Check sheet for the modelled part. Datum: model origin and axes. Units: mm. Face numbers are marked on the shaded views. A direction names the side the tool comes from. Coordinates: 2 decimals unless noted, no trailing zeros. Loops run counter-clockwise (first coordinate to the right, second up) from the corner with the lowest first, then second, coordinate; pieces in that order, holes last.
from build123d import *

# Parameters (mm, degrees)
SKETCH_1_R               = 25
SKETCH_1_R_2             = 1.5
EXTRUDE_1_DEPTH          = 2.5
CUT_EXTRUDE_2_DEPTH      = 36.443617197
CUT_EXTRUDE_2_DEPTH_BACK = 36.443617197
SKETCH_3_R               = 4
CUT_EXTRUDE_5_DEPTH      = 10
FILLET_2_R               = 3
EXTRUDE_2_DEPTH          = 10


with BuildPart() as part:
    # 草图1 → 凸台-拉伸1 (new body)
    with BuildSketch(Plane.XY):
        Circle(SKETCH_1_R)
        with Locations((0, 22)):
            Circle(SKETCH_1_R_2, mode=Mode.SUBTRACT)
        with Locations((22, 0)):
            Circle(SKETCH_1_R_2, mode=Mode.SUBTRACT)
        with Locations((0, -22)):
            Circle(SKETCH_1_R_2, mode=Mode.SUBTRACT)
        with Locations(Location((-22, 0, 0), (0, 0, 180))):
            Circle(SKETCH_1_R_2, mode=Mode.SUBTRACT)
    extrude(amount=EXTRUDE_1_DEPTH)

    # 草图3 → 切除-拉伸2 (cut, two sides: drawn at the far end of the back side and taken through both)
    with BuildSketch(Plane(origin=(0, 0, 0), x_dir=(-1, 0, 0), z_dir=(0, 0, -1)).offset(-CUT_EXTRUDE_2_DEPTH_BACK)):
        Circle(SKETCH_3_R)
    extrude(amount=CUT_EXTRUDE_2_DEPTH + CUT_EXTRUDE_2_DEPTH_BACK, mode=Mode.SUBTRACT)

    # 草图5 → 切除-拉伸5 (cut)
    with BuildSketch(Plane(origin=(0, 0, 0), x_dir=(-1, 0, 0), z_dir=(0, 0, -1))):
        with BuildLine():
            ThreePointArc((-2.638187412, 24.860409634), (-17.67766953, 17.67766953), (-24.860409634, 2.638187412))
            ThreePointArc((-24.860409634, 2.638187412), (-10.606601718, 10.606601718), (-2.638187412, 24.860409634))
        make_face()
        with BuildLine():
            ThreePointArc((-2.638187412, -24.860409634), (-10.606601718, -10.606601718), (-24.860409634, -2.638187412))
            ThreePointArc((-24.860409634, -2.638187412), (-17.67766953, -17.67766953), (-2.638187412, -24.860409634))
        make_face()
        with BuildLine():
            ThreePointArc((24.860409634, -2.638187412), (10.606601718, -10.606601718), (2.638187412, -24.860409634))
            ThreePointArc((2.638187412, -24.860409634), (17.67766953, -17.67766953), (24.860409634, -2.638187412))
        make_face()
        with BuildLine():
            ThreePointArc((24.860409634, 2.638187412), (17.67766953, 17.67766953), (2.638187412, 24.860409634))
            ThreePointArc((2.638187412, 24.860409634), (10.606601718, 10.606601718), (24.860409634, 2.638187412))
        make_face()
    extrude(amount=-CUT_EXTRUDE_5_DEPTH, mode=Mode.SUBTRACT)

    # 圆角2
    fillet_2_edges = [part.edges().sort_by_distance(p)[0] for p in [
        (2.638187412, 24.860409634, 1.25),
        (24.860409634, 2.638187412, 1.25),
        (24.860409634, -2.638187412, 1.25),
        (2.638187412, -24.860409634, 1.25),
        (-2.638187412, -24.860409634, 1.25),
        (-24.860409634, -2.638187412, 1.25),
        (-24.860409634, 2.638187412, 1.25),
        (-2.638187412, 24.860409634, 1.25),
    ]]
    fillet(fillet_2_edges, radius=FILLET_2_R)

    # 草图6 → 凸台-拉伸2 (add)
    with BuildSketch(Plane.XY.offset(2.5)):
        with BuildLine():
            Line((-11.761483572, 2.380652052), (-2.380652052, 11.761483572))
            ThreePointArc((-2.380652052, 11.761483572), (8.485281374, 8.485281374), (11.761483572, -2.380652052))
            Line((11.761483572, -2.380652052), (2.380652052, -11.761483572))
            ThreePointArc((2.380652052, -11.761483572), (-8.485281374, -8.485281374), (-11.761483572, 2.380652052))
        make_face()
        with BuildLine():
            Line((-10.163012909, 0.867852878), (-0.867852878, 10.163012909))
            ThreePointArc((-0.867852878, 10.163012909), (7.212489168, 7.212489168), (10.163012909, -0.867852878))
            Line((10.163012909, -0.867852878), (0.867852878, -10.163012909))
            ThreePointArc((0.867852878, -10.163012909), (-7.212489168, -7.212489168), (-10.163012909, 0.867852878))
        make_face(mode=Mode.SUBTRACT)
    extrude(amount=EXTRUDE_2_DEPTH)


solid = part.part
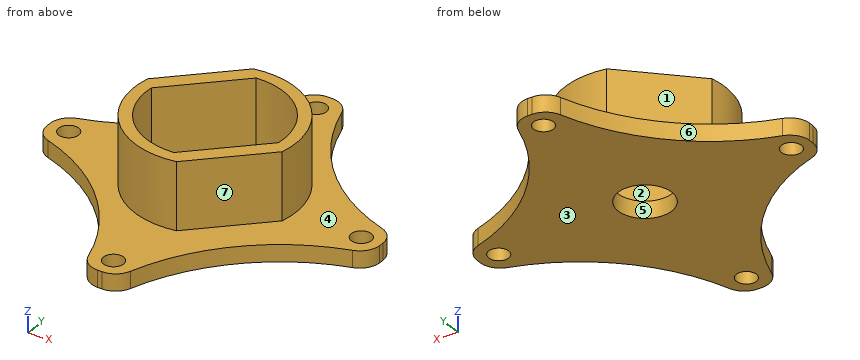
(1) Section check D-D, the plane x = -6. Enter the section's corners in (y, z).
(2) Gauge pin test, flat ends, axial feed: P1, Ø1.5, axis at y = -4, z = 8.5, coming from the +X side; P2, Ø9, axis at x = 0, y = 0, coming from the +Z side; P3, Ø2, axis at y = 8, z = 5, coming from the -X side. Record the tip position at first contact, or that the pin passes through.
(3) Section check B-B, the plane y = 22. Enter the section's corners in (x, z), plus the area to 3 significant figures.
(4) Draft check along Y on the marked faces 4, 5, 6 and 7. Enter one of: pulls with the +Y half, pulls with the -Y half, needs draft (parallel to the pull), parting line crosses it, or undercut.
(5) Set-up check for the marked faces 1, 2 and 3: record each of +Z, -Z, +X, -X, +Y, -Y from which the full face is reachable in a straight line by a thin tool's end or side.
(6) Scan lines: line 1 along Y through (x, z) = (0, 0.8); line 2 along Y through (x, z) = (0, 4); line 3 along Z through (x, y) = (-9, 2). Record each from-to range of solid material in increasing order.
(7) Section check A-A, the plane z = 6. Enter the section's corners in (x, y), plus the area to 3 significant figures.
Determined:
1. outline: (-16.54, 0) - (16.54, 0) - (16.54, 2.5) - (8.14, 2.5) - (8.14, 12.5) - (5.03, 12.5) - (5.03, 2.5) - (-8.25, 2.5) - (-8.25, 12.5) - (-10.39, 12.5) - (-10.39, 2.5) - (-16.54, 2.5) - close
2. P1: stops at x = 10.89
2. P2: stops at z = 2.5
2. P3: stops at x = -7.14
3. outline: (-3.47, 0) - (-1.5, 0) - (-1.5, 2.5) - (-3.47, 2.5) - close; (1.5, 0) - (3.47, 0) - (3.47, 2.5) - (1.5, 2.5) - close
3. area: 9.86 mm2
4. face 4: needs draft
4. face 5: undercut
4. face 6: pulls with the +Y half
4. face 7: pulls with the -Y half
5. face 1: +Z, -X, +Y
5. face 2: +Z
5. face 3: -Z, +X, -X, +Y, -Y
6. line 1: y = -25 to -23.5, -20.5 to -4, 4 to 20.5, 23.5 to 25
6. line 2: y = -12 to -10.2, 10.2 to 12
6. line 3: z = 0 to 2.5
7. outline: (-11.76, 2.38) arc R12 ccw to (2.38, -11.76) - (11.76, -2.38) arc R12 ccw to (-2.38, 11.76) - close; hole (-10.16, 0.87) arc R10.2 ccw to (0.87, -10.16) - (10.16, -0.87) arc R10.2 ccw to (-0.87, 10.16) - close
7. area: 133 mm2
